```python
from build123d import *

# Parameters (mm, degrees)
BOSS_EXTRUDE1_DEPTH = 8
SKETCH2_R           = 2
BOSS_EXTRUDE2_DEPTH = 8
SKETCH3_R           = 1.5
CUT_EXTRUDE1_DEPTH  = 15


with BuildPart() as part:
    # Sketch1 → Boss-Extrude1 (new body)
    with BuildSketch(Plane(origin=(0, 0, 0), x_dir=(0, 0, -1), z_dir=(1, 0, 0))):
        with BuildLine():
            Line((17, 0), (20, 0))
            Line((20, 0), (20, -5))
            Line((20, -5), (0, -5))
            Line((0, -5), (0, 0))
            Line((0, 0), (3, 0))
            ThreePointArc((3, 0), (10, 7), (17, 0))
        make_face()
    extrude(amount=BOSS_EXTRUDE1_DEPTH)

    # Sketch2 → Boss-Extrude2 (add)
    with BuildSketch(Plane(origin=(8, 0, 0), x_dir=(0, 0, -1), z_dir=(1, 0, 0))):
        with Locations((10, 0)):
            Circle(SKETCH2_R)
    extrude(amount=BOSS_EXTRUDE2_DEPTH)

    # Sketch3 → Cut-Extrude1 (cut)
    with BuildSketch(Plane.XZ.offset(5)):
        with Locations(Location((3, -5, 0), (0, 0, 270))):
            Circle(SKETCH3_R)
        with Locations(Location((3, -15, 0), (0, 0, 270))):
            Circle(SKETCH3_R)
    extrude(amount=-CUT_EXTRUDE1_DEPTH, mode=Mode.SUBTRACT)


solid = part.part
```
Work out the finished part from the listing and answer in its coordinate system (mm). A direction names the side the tool comes from. Give positions to 0.01 mm unless a question says otherwise; leave off trailing zeros. Write each loop counter-clockwise with the first axis right and the second up, starting at its lowest first coordinate (ties: lowest second). Pieces come first, ordered by that corner, then holes. Notation, with made-up numbers: (67, 68.25) -> (114, 68.25) arc R15 cw to (114, 75.25) -> close; hole circle Ø6 at (56.25, 15). An arc over 180 degrees is marked (long way). Write each question's results on one line, items separated by ' | '.
1. Straight lines are drawn through the part: L1, parallel to Z at x = 3, y = 0.25; L2, parallel to X at y = 3.25, z = -15; L3, parallel to Z at x = 3.25, y = -2.5. For each, find the intervals that lie inside material, in ascending order.
Data:
L1: -17 to -16.5, -13.5 to -6.5, -3.5 to -3 | L2: 0 to 1.5, 4.5 to 8 | L3: -20 to -16.48, -13.52 to -6.48, -3.52 to 0
2. Each of these flat-tipped pins is pushed along its axis until it touches: pin 1 Ø5 at (x, y) = (2, 4) entering from +Z; pin 2 Ø1.5 at (y, z) = (4, -12.5) entering from +X; pin 3 Ø0.9 at (x, z) = (3.5, -2) entering from +Y. Where does it stop, or does it pass through?
Data:
pin 1: z = -3.16 | pin 2: x = 8 | pin 3: y = 0
3. Determine the mould class of faces 1 (the flat face through (4, -3, 0)), 2 (the cylindrical face through (3.07, -0.78, -13.5)), 3 (the flat face through (16, 0, -10)), 4 (the flat face through (0, 0, -10)) for opening direction X: +X half, -X half, draft (parallel to the pull), parting line (faces both ways), or undercut.
Data:
face 1: draft | face 2: undercut | face 3: +X half | face 4: -X half
4. Find section B-B on z = -5. Determine the outline of the cut face in (x, y).
Data:
outline: (0, -5) -> (1.5, -5) -> (1.5, 4.9) -> (0, 4.9) -> close; (4.5, -5) -> (8, -5) -> (8, 4.9) -> (4.5, 4.9) -> close
5. A tool of negligible diameter and unlimited length cuts with its end or side. For faces 5 (the flat face through (4, -5, -10)), 6 (the flat face through (4, 0, -1)), 7 (the cylindrical face through (11.9, -1.2, -8.4)), 8 (the flat face through (4, 0, -18)), from which of +Z, -Z, +X, -X, +Y, -Y can it reach the whole face along a straight path? Write none if from no direction.
Data:
face 5: +Z, -Z, +X, -X, -Y | face 6: +Z, +X, -X, +Y | face 7: +X | face 8: -Z, +X, -X, +Y
6. Find section A-A on x = 4.25. Determine the outline of the cut face in (y, z), and give its area (3 significant figures).
Data:
outline: (-5, -20) -> (0, -20) -> (0, -17) arc R7 ccw to (3.88, -15.83) -> (-5, -15.83) -> close; (-5, -14.17) -> (5.62, -14.17) arc R7 ccw to (5.62, -5.83) -> (-5, -5.83) -> close; (-5, -4.17) -> (3.88, -4.17) arc R7 ccw to (0, -3) -> (0, 0) -> (-5, 0) -> close | area: 144 mm^2
7. Find section C-C on y = -0.75. Determine the outline of the cut face in (x, z), and give its area (3 significant figures).
Data:
outline: (0, -20) -> (8, -20) -> (8, -11.85) -> (16, -11.85) -> (16, -8.15) -> (8, -8.15) -> (8, 0) -> (0, 0) -> close; hole circle Ø3 at (3, -15); hole circle Ø3 at (3, -5) | area: 176 mm^2
8. Find section D-D on x = 6.75. Determine the outline of the cut face in (y, z).
Data:
outline: (-5, -20) -> (0, -20) -> (0, -17) arc R7 ccw to (0, -3) -> (0, 0) -> (-5, 0) -> close
